The listing builds one solid part. Answer for the finished solid, in the listing's coordinates (mm). A direction names the side the tool comes from. Coordinates: 2 decimals unless noted, no trailing zeros. Loops run counter-clockwise (first coordinate to the right, second up) from the corner with the lowest first, then second, coordinate; pieces in that order, holes last. Notation, with made-up numbers: (-7, 57.25) - (3, 57.25) arc R21 cw to (3, 96.25) - close; hole circle Ø10 at (52, -30.5). An arc over 180 degrees is marked (long way). Return JSON: item names as keys, results as strings. Group by question number.
1. Section C-C (x = 174) is taken. Write down the section's boundary in (y, z), and give its area (3 significant figures).
2. Each of these flat-tipped pins is pushed along its axis until it touches: P1, Ø7, axis at x = -95, y = -335, coming from the -Z side; P2, Ø3, axis at y = -367.5, z = 12, coming from the +X side; P3, Ø9, axis at x = 313.5, z = 9.5, coming from the +Y side; P4, Ø6, axis at x = 294, z = 8.5, coming from the -Y side. Where does it stop, or does it pass through?
3. Find the intervals of material crossed by line 1 along X through (y, z) = (-265, 4.5); line 2 along X through (y, z) = (-335, 10.5); line 3 along Y through (x, z) = (275, 4.5), in increasing order.
4. Section A-A (y = -345) is taken. Write down the section's boundary in (x, z).
5. Section B-B (z = 3) is taken. Write down the section's boundary in (x, y), and give its area (3 significant figures).
6. The mould has two halves that part along X. Classify faces 6 (the face through (109, -343, 15)), 7 (the face through (355, -346, 7)), 8 (the face through (-21, -465, 7)): pulls with the +X half, pulls with the -X half, needs draft (parallel to the pull), parting line crosses it, or undercut.
7. Which of the six approach directions +Z, -Z, +X, -X, +Y, -Y give full straight-line access (tool end or side, diameter ignored) to faces 1 (the face through (229, -465, 7)), 2 (the face through (231, -225, 7)), 3 (the face through (-145, -344, 7)), 4 (the face through (319, -305, 7)), 5 (the face through (109, -343, 0))?
8. Section D-D (y = -275) is taken. Write down the section's boundary in (x, z).
```python
from build123d import *

# Parameters (mm, degrees)
F1_DEPTH = 15
F2_R     = 15
F2_W     = 12
F2_H     = 8
F2_R_2   = 6.5
F2_R_3   = 4
F2_R_4   = 2
F3_DEPTH = 40
F4_ANGLE = 90


with BuildPart() as f1:
    # F0 (on Top) → F1 (new body)
    with BuildSketch(Plane.XY):
        with BuildLine():
            Line((-120, 225), (-120, 250))
            Line((-120, 250), (-95, 250))
            ThreePointArc((-95, 250), (-137.6776695297, 267.6776695297), (-120, 225))
        make_face()
        with BuildLine():
            Line((-95, 250), (-120, 250))
            Line((-120, 250), (-120, 225))
            ThreePointArc((-120, 225), (-102.3223304703, 232.3223304703), (-95, 250))
        make_face()
        with BuildLine():
            Line((95, 250), (-95, 250))
            ThreePointArc((-95, 250), (-102.3223304703, 232.3223304703), (-120, 225))
            Line((-120, 225), (-120, 25))
            ThreePointArc((-120, 25), (-102.3223304703, 17.6776695297), (-95, 0))
            ThreePointArc((-95, 0), (-102.3223304703, -17.6776695297), (-120, -25))
            Line((-120, -25), (-120, -225))
            ThreePointArc((-120, -225), (-102.3223304703, -232.3223304703), (-95, -250))
            Line((-95, -250), (95, -250))
            ThreePointArc((95, -250), (102.3223304703, -232.3223304703), (120, -225))
            Line((120, -225), (120, -25))
            ThreePointArc((120, -25), (95, 0), (120, 25))
            Line((120, 25), (120, 225))
            ThreePointArc((120, 225), (102.3223304703, 232.3223304703), (95, 250))
        make_face()
        with BuildLine():
            ThreePointArc((145, 250), (120, 275), (95, 250))
            Line((95, 250), (120, 250))
            Line((120, 250), (120, 225))
            ThreePointArc((120, 225), (137.6776695297, 232.3223304703), (145, 250))
        make_face()
        with BuildLine():
            Line((120, 250), (95, 250))
            ThreePointArc((95, 250), (102.3223304703, 232.3223304703), (120, 225))
            Line((120, 225), (120, 250))
        make_face()
        with BuildLine():
            ThreePointArc((-95, 0), (-102.3223304703, 17.6776695297), (-120, 25))
            Line((-120, 25), (-120, -25))
            ThreePointArc((-120, -25), (-102.3223304703, -17.6776695297), (-95, 0))
        make_face()
        with BuildLine():
            Line((-120, -25), (-120, 25))
            ThreePointArc((-120, 25), (-145, 0), (-120, -25))
        make_face()
        with BuildLine():
            ThreePointArc((145, 0), (137.6776695297, 17.6776695297), (120, 25))
            Line((120, 25), (120, -25))
            ThreePointArc((120, -25), (137.6776695297, -17.6776695297), (145, 0))
        make_face()
        with BuildLine():
            Line((120, -25), (120, 25))
            ThreePointArc((120, 25), (95, 0), (120, -25))
        make_face()
        with BuildLine():
            ThreePointArc((-95, -250), (-102.3223304703, -232.3223304703), (-120, -225))
            Line((-120, -225), (-120, -250))
            Line((-120, -250), (-95, -250))
        make_face()
        with BuildLine():
            Line((-120, -250), (-120, -225))
            ThreePointArc((-120, -225), (-137.6776695297, -267.6776695297), (-95, -250))
            Line((-95, -250), (-120, -250))
        make_face()
        with BuildLine():
            ThreePointArc((145, -250), (137.6776695297, -232.3223304703), (120, -225))
            Line((120, -225), (120, -250))
            Line((120, -250), (95, -250))
            ThreePointArc((95, -250), (120, -275), (145, -250))
        make_face()
        with BuildLine():
            Line((120, -250), (120, -225))
            ThreePointArc((120, -225), (102.3223304703, -232.3223304703), (95, -250))
            Line((95, -250), (120, -250))
        make_face()
    extrude(amount=F1_DEPTH)

    # F2 (on face) → F3 (cut)
    with BuildSketch(Plane(origin=(0, 0, 0), x_dir=(1, 0, 0), z_dir=(0, 0, -1))):
        with Locations((0, -210)):
            Circle(F2_R)
        with Locations((-40, -210)):
            Rectangle(F2_W, F2_H)
        with Locations((-70, -210)):
            Circle(F2_R_2)
        with Locations((-90, -210)):
            Circle(F2_R_2)
        with Locations((-10, 200)):
            Circle(F2_R_3)
        with Locations((-80, -170)):
            Circle(F2_R_4)
    extrude(amount=-F3_DEPTH, mode=Mode.SUBTRACT)


with BuildPart() as f1_1:
    # F4: moved
    add(f1.part.rotate(Axis((-120, -225, 7.5), (0, 0, -1)), F4_ANGLE))


solid = f1_1.part
```
The answers:
{
 "1": {"outline": "(-465, 0) - (-225, 0) - (-225, 15) - (-465, 15) - close", "area": "3,600 mm2"},
 "2": {"P1": "passes through", "P2": "stops at x = 355", "P3": "stops at y = -225", "P4": "stops at y = -465"},
 "3": {"line 1": "x = -145 to 273, 277 to 355", "line 2": "x = -145 to -99, -91 to 303.82, 326.18 to 355", "line 3": "y = -465 to -267, -263 to -225"},
 "4": {"outline": "(-145, 0) - (300, 0) - (300, 15) - (-145, 15) - close; (330, 0) - (355, 0) - (355, 15) - (330, 15) - close"},
 "5": {"outline": "(-145, -440) arc R25 ccw (long way) to (-120, -465) - (80, -465) arc R25 ccw to (130, -465) - (330, -465) arc R25 ccw (long way) to (355, -440) - (355, -250) arc R25 ccw (long way) to (330, -225) - (130, -225) arc R25 ccw to (80, -225) - (-120, -225) arc R25 ccw (long way) to (-145, -250) - close; hole circle Ø8 at (-95, -335); hole circle Ø4 at (275, -265); hole circle Ø30 at (315, -345); hole circle Ø13 at (315, -275); hole circle Ø13 at (315, -255); hole (311, -311) - (319, -311) - (319, -299) - (311, -299) - close", "area": "127,000 mm2"},
 "6": {"face 6": "needs draft", "face 7": "pulls with the +X half", "face 8": "undercut"},
 "7": {"face 1": "+Z, -Z, -Y", "face 2": "+Z, -Z, +Y", "face 3": "+Z, -Z, -X", "face 4": "+Z, -Z", "face 5": "-Z, +X, -X, +Y, -Y"},
 "8": {"outline": "(-145, 0) - (308.5, 0) - (308.5, 15) - (-145, 15) - close; (321.5, 0) - (355, 0) - (355, 15) - (321.5, 15) - close"}
}
